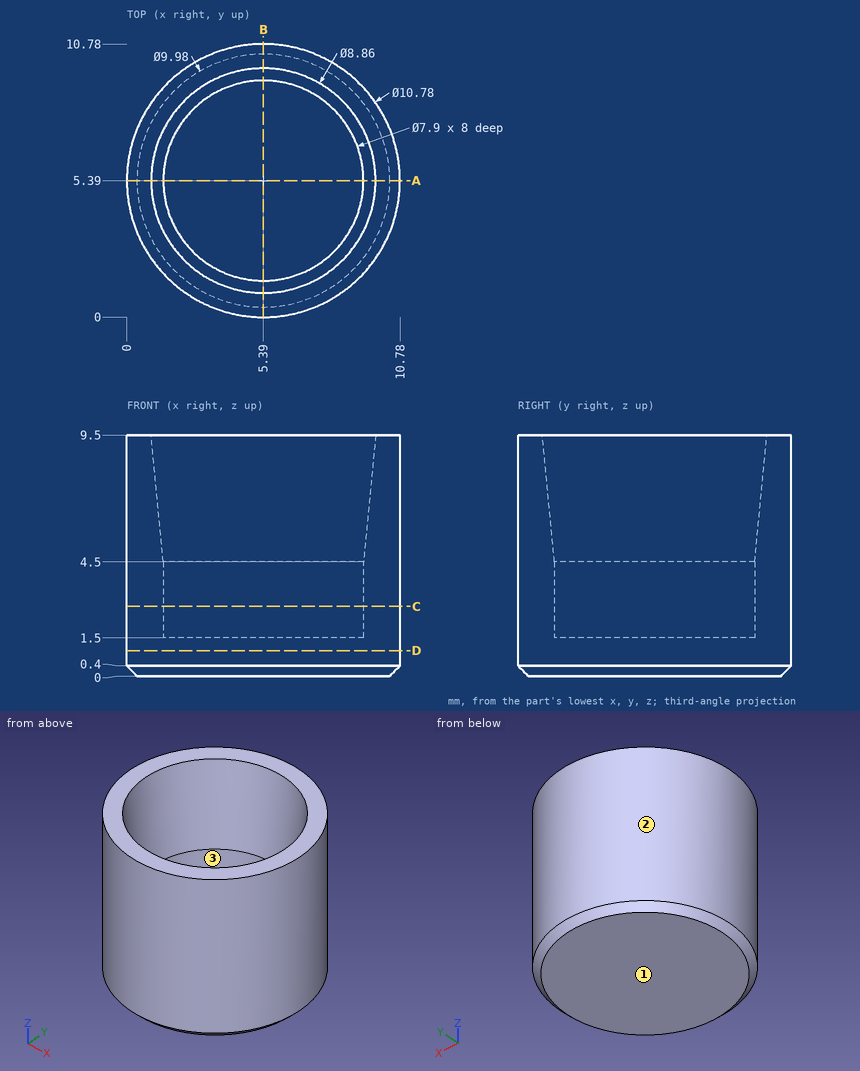
Part print with two shaded views. Sizes in mm from the minimum x, y, z corner. Give positions to 0.01 mm unless a question says otherwise; leave off trailing zeros. Order: outer loops, then holes, each group sorted by start corner. A loop starts at its lowest first (then second) coordinate and runs counter-clockwise, first axis right, second up. Notation, with made-up numbers: M 75,35.5 L 83,35.5 A15 cw 83,57.5 Z; hole C -7.75,44.5 d8. An arc over 180 degrees is marked long. Put each result on its own line as item: value.
Item 1: Pull direction X, two halves, no side cores. Call the marked faces 1, 2 and 3: +X half, -X half, draft (parallel to the pull), parting line (faces both ways), or undercut.
Results are:
face 1: draft
face 2: parting line
face 3: undercut
Item 2: Drop flat-ended pins along their axis: pin 1 Ø1.5 at (x, z) = (8, 3.5) entering from +Y; pin 2 Ø1.5 at (y, z) = (2.5, 3) entering from -X; pin 3 Ø4 at (x, y) = (3.5, 5.5) entering from +Z. Give the stop position or say it passes through.
Results are:
pin 1: y = 10.45
pin 2: x = 0.44
pin 3: z = 1.5
Item 3: Cut at D-D on z = 1. Write the cut outline in (x, y), then the cut area to 3 significant figures.
Results are:
outline: C 5.39,5.39 d10.78
area: 91.3 mm2
Item 4: Wall check: probe 1 along Y at (x, z) = (5.39, 3.8); probe 2 along Z at (x, y) = (8, 4.5); probe 3 along Y at (x, z) = (4.25, 3). Give the ranges that are in metal, low to high.
Results are:
probe 1: 0 to 1.44, 9.34 to 10.78
probe 2: 0 to 1.5
probe 3: 0.12 to 1.61, 9.17 to 10.66
Item 5: Cut at A-A on y = 5.39. Write the cut outline in (x, z), then the cut area to 4 significant figures.
Results are:
outline: M 0,0.4 L 0.4,0 L 10.38,0 L 10.78,0.4 L 10.78,9.5 L 9.82,9.5 L 9.34,4.5 L 9.34,1.5 L 1.44,1.5 L 1.44,4.5 L 0.96,9.5 L 0,9.5 Z
area: 36.65 mm2
Item 6: Cut at C-C on z = 2.75. Write the cut outline in (x, y), then the cut area to 3 significant figures.
Results are:
outline: C 5.39,5.39 d10.78; hole C 5.39,5.39 d7.9
area: 42.3 mm2
